```python
from build123d import *

# Parameters (mm, degrees)
F0_R     = 10
F0_R_2   = 6
F1_DEPTH = 13
F2_R     = 12
F2_R_2   = 6
F3_DEPTH = 1.5
F4_R     = 9.25
F4_R_2   = 6
F5_DEPTH = 5


with BuildPart() as f1:
    # F0 (on Top) → F1 (new body)
    with BuildSketch(Plane.XY):
        Circle(F0_R)
        Circle(F0_R_2, mode=Mode.SUBTRACT)
    extrude(amount=F1_DEPTH)

    # F2 (on face) → F3 (join)
    with BuildSketch(Plane.XY.offset(13)):
        Circle(F2_R)
        Circle(F2_R_2, mode=Mode.SUBTRACT)
    extrude(amount=F3_DEPTH)

    # F4 (on face) → F5 (cut)
    with BuildSketch(Plane.XY.offset(14.5)):
        Circle(F4_R)
        Circle(F4_R_2, mode=Mode.SUBTRACT)
    extrude(amount=-F5_DEPTH, mode=Mode.SUBTRACT)


solid = f1.part
```
Source: CAD feature listing. Evaluate the final solid. Frame: model axes, mm. A direction names the side the tool comes from. Coordinates: 2 decimals unless noted, no trailing zeros. Order: outer loops, then holes, each group sorted by start corner. A loop starts at its lowest first (then second) coordinate and runs counter-clockwise, first axis right, second up. Notation, with made-up numbers: (24.25, 36.5) - (58.25, 36.5) arc R30 ccw to (58.25, 75.5) - close; hole circle Ø11 at (-1, 64). An arc over 180 degrees is marked (long way). One line per item, written item: value.
1) Reachability of faces 1 (the face through (2, -6, 9.5)), 2 (the face through (-6, 0, 5)), 3 (the face through (-2.17, -9.76, 6.41)) from +Z, -Z, +X, -X, +Y, -Y: full face, straight path, thin tool, end or side. Return the list, or none.
Computed values:
face 1: +Z
face 2: +Z, -Z
face 3: -Z
2) Contact query for flat-ended pins moving along their axis: pin 1 (1 mm diameter, centred on x = -1.5, z = 9, fed in from +Y); pin 2 (6 mm diameter, centred on x = -4, z = 6, fed in from -Y); pin 3 (2 mm diameter, centred on x = 9, z = 10.5, fed in from -Y); pin 4 (11 mm diameter, centred on x = 0, y = 0, fed in from -Z). Output: stop coordinate, or through.
Computed values:
pin 1: stops at y = 9.95
pin 2: stops at y = -9.95
pin 3: stops at y = -6
pin 4: passes through
3) Cut plane C-C on z = 12. Output: boundary loops of the cut face in (x, y).
Computed values:
outline: circle Ø20 at (0, 0); hole circle Ø18.5 at (0, 0)
4) Cut plane D-D on y = 6.5. Output: boundary loops of the cut face in (x, z).
Computed values:
outline: (-10.09, 13) - (-7.6, 13) - (-7.6, 0) - (7.6, 0) - (7.6, 13) - (10.09, 13) - (10.09, 14.5) - (6.58, 14.5) - (6.58, 9.5) - (-6.58, 9.5) - (-6.58, 14.5) - (-10.09, 14.5) - close
5) Mould query, pull axis X, two halves, no side actions, for faces 4 (the face through (0, -7, 0)), 5 (the face through (-11.99, 0.53, 13.74)), 6 (the face through (-2.01, -9.03, 12.04)). Classes: released by +X, released by -X, zero draft, split by the parting line, or undercut.
Computed values:
face 4: zero draft
face 5: split by the parting line
face 6: undercut
6) Ray query, line 1 (Y direction, x = 0, z = 13.2); line 2 (Y direction, x = 0, z = 5.25); line 3 (Z direction, x = 7, y = 2). Return the intervals inside material, ascending. Write a range as [from, to].
Computed values:
line 1: y = [-12, -9.25], [9.25, 12]
line 2: y = [-10, -6], [6, 10]
line 3: z = [0, 9.5]
7) Cut plane A-A on y = 0. Output: boundary loops of the cut face in (x, z), plus the area to 3 significant figures.
Computed values:
outline: (-12, 13) - (-10, 13) - (-10, 0) - (-6, 0) - (-6, 9.5) - (-9.25, 9.5) - (-9.25, 14.5) - (-12, 14.5) - close; (6, 0) - (10, 0) - (10, 13) - (12, 13) - (12, 14.5) - (9.25, 14.5) - (9.25, 9.5) - (6, 9.5) - close
area: 89.5 mm^2
8) Cut plane B-B on x = 3.5. Output: boundary loops of the cut face in (y, z), plus the area to 3 significant figures.
Computed values:
outline: (-11.48, 13) - (-9.37, 13) - (-9.37, 0) - (-4.87, 0) - (-4.87, 9.5) - (-8.56, 9.5) - (-8.56, 14.5) - (-11.48, 14.5) - close; (4.87, 0) - (9.37, 0) - (9.37, 13) - (11.48, 13) - (11.48, 14.5) - (8.56, 14.5) - (8.56, 9.5) - (4.87, 9.5) - close
area: 99.8 mm^2
